Check sheet for the modelled part. Datum: model origin and axes. Units: mm. Coordinates: 2 decimals unless noted, no trailing zeros. Loops run counter-clockwise (first coordinate to the right, second up) from the corner with the lowest first, then second, coordinate; pieces in that order, holes last. Notation, with made-up numbers: (38.5, 40.5) -> (73.5, 40.5) arc R19 ccw to (73.5, 55.5) -> close; hole circle Ø4 at (48, 61.5). An arc over 180 degrees is marked (long way). Use one line per item in the form item = value.
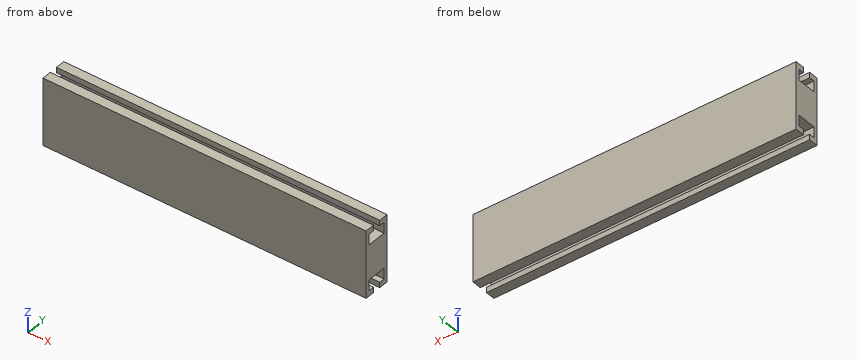
from build123d import *

# Parameters (mm, degrees)
SKETCH1_W           = 120
SKETCH1_H           = 25
BOSS_EXTRUDE1_DEPTH = 10
CUT_EXTRUDE1_DEPTH  = 120
CUT_EXTRUDE2_DEPTH  = 120


with BuildPart() as part:
    # Sketch1 → Boss-Extrude1 (new body)
    with BuildSketch(Plane(origin=(0, 0, 0), x_dir=(1, 0, 0), z_dir=(0, 1, 0))):
        with Locations((-95.061127507, -76.27261395)):
            Rectangle(SKETCH1_W, SKETCH1_H)
    extrude(amount=BOSS_EXTRUDE1_DEPTH)

    # Sketch2 → Cut-Extrude1 (cut)
    with BuildSketch(Plane(origin=(-35.061127507, 0, 0), x_dir=(0, 0, -1), z_dir=(1, 0, 0))):
        Polygon((-63.77261395, 6.5), (-65.77261395, 6.5), (-65.77261395, 8.55), (-69.77261395, 8.55), (-69.77261395, 1.45), (-65.77261395, 1.45), (-65.77261395, 3.5), (-63.77261395, 3.5), align=None)
    extrude(amount=-CUT_EXTRUDE1_DEPTH, mode=Mode.SUBTRACT)

    # Sketch3 → Cut-Extrude2 (cut)
    with BuildSketch(Plane(origin=(-35.061127507, 0, 0), x_dir=(0, 0, -1), z_dir=(1, 0, 0))):
        Polygon((-88.77261395, 6.5), (-86.77261395, 6.5), (-86.77261395, 8.55), (-82.77261395, 8.55), (-82.77261395, 1.45), (-86.77261395, 1.45), (-86.77261395, 3.5), (-88.77261395, 3.5), align=None)
    extrude(amount=-CUT_EXTRUDE2_DEPTH, mode=Mode.SUBTRACT)


solid = part.part
(1) Scan lines: line 1 along Z through (x, y) = (-45, 8.5); line 2 along Y through (x, z) = (-143, 65.5); line 3 along Y through (x, z) = (-60.5, 68). Record each from-to range of solid material in increasing order.
Established:
line_1 = 63.77 to 65.77, 69.77 to 82.77, 86.77 to 88.77
line_2 = 0 to 3.5, 6.5 to 10
line_3 = 0 to 1.45, 8.55 to 10
(2) Section check A-A, the plane z = 67.25. Record the boundary of the cut face in (x, y), plus the area to 3 significant figures.
Established:
outline = (-155.06, 0) -> (-35.06, 0) -> (-35.06, 1.45) -> (-155.06, 1.45) -> close; (-155.06, 8.55) -> (-35.06, 8.55) -> (-35.06, 10) -> (-155.06, 10) -> close
area = 348 mm²
(3) Section check B-B, the plane x = -134.5. Record the boundary of the cut face in (y, z), plus the area to 3 significant figures.
Established:
outline = (0, 63.77) -> (3.5, 63.77) -> (3.5, 65.77) -> (1.45, 65.77) -> (1.45, 69.77) -> (8.55, 69.77) -> (8.55, 65.77) -> (6.5, 65.77) -> (6.5, 63.77) -> (10, 63.77) -> (10, 88.77) -> (6.5, 88.77) -> (6.5, 86.77) -> (8.55, 86.77) -> (8.55, 82.77) -> (1.45, 82.77) -> (1.45, 86.77) -> (3.5, 86.77) -> (3.5, 88.77) -> (0, 88.77) -> close
area = 181 mm²
(4) Go/stop test with a flat-tipped pin: P1, Ø1.5, axis at x = -57, y = 4.5, coming from the +Z side. Record where the tip stops, or that it passes through.
Established:
P1 = 82.77
